Drawing for the job (mm, zero at the part's lowest x, y, z). Give positions to 0.01 mm unless a question says otherwise; leave off trailing zeros. Order: outer loops, then holes, each group sorted by start corner. A loop starts at its lowest first (then second) coordinate and runs counter-clockwise, first axis right, second up. Notation, with made-up numbers: (53, -15.75) - (59, -15.75) arc R7 ccw to (59, -10.75) - close; hole circle Ø5 at (-32.75, -1.75). An arc over 180 degrees is marked (long way). One line per item, written item: value.
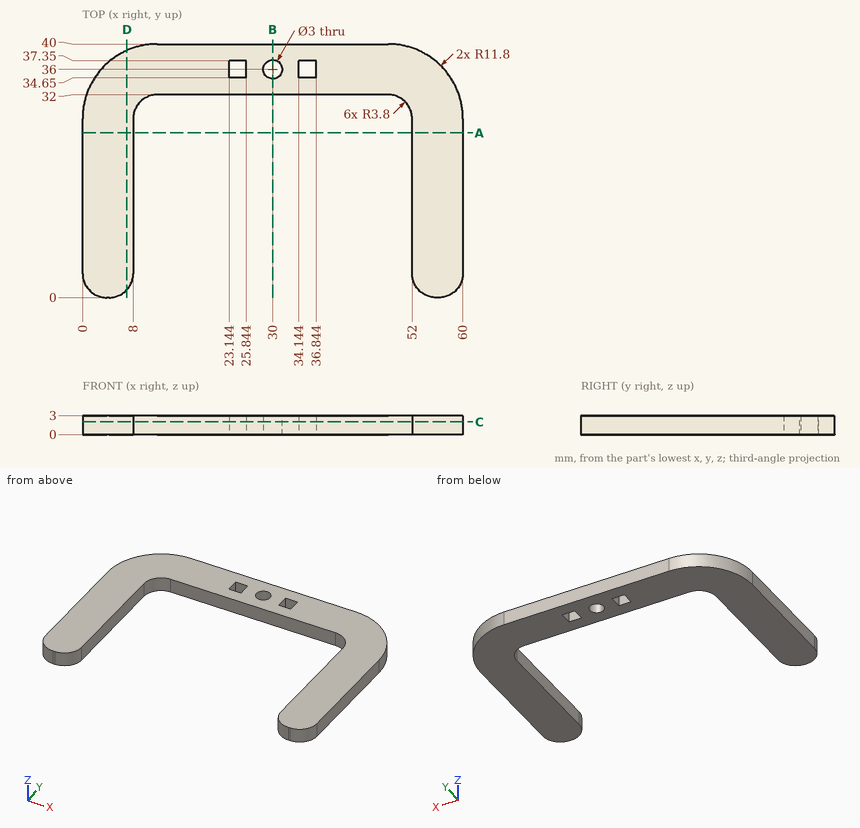
1) Cut at B-B, the plane x = 30. Give the cut face in (y, z).
Outcome:
outline: (32, 0) - (34.5, 0) - (34.5, 3) - (32, 3) - close; (37.5, 0) - (40, 0) - (40, 3) - (37.5, 3) - close
2) Cut at D-D, the plane x = 7. Give the cut face in (y, z).
Outcome:
outline: (1.23, 0) - (38.98, 0) - (38.98, 3) - (1.23, 3) - close
3) Cut at C-C, the plane z = 2. Give the number of separate pieces and of enclosed holes in the cut face.
Outcome:
separate pieces: 1
enclosed holes: 3
4) Drill centre lines: line 1 along Y through (x, z) = (30, 1.6); line 2 along X through (y, z) = (23.5, 1.8); line 3 along X through (y, z) = (36, 2.3) (1 decimal). Where is each one in solid material? Low to high. Write a range as from..to.
Outcome:
line 1: y = 32..34.5, 37.5..40
line 2: x = 0..8, 52..60
line 3: x = 2.9..23.1, 25.8..28.5, 31.5..34.1, 36.8..57.1
5) Cut at A-A, the plane y = 26. Give the cut face in (x, z).
Outcome:
outline: (0, 0) - (8, 0) - (8, 3) - (0, 3) - close; (52, 0) - (60, 0) - (60, 3) - (52, 3) - close
6) Pin check, flat tips, straight feed: pin 1 (0.8 mm diameter, centred on y = 35.5, z = 2, fed in from +X); pin 2 (1.5 mm diameter, centred on x = 23.5, z = 1.5, fed in from -Y); pin 3 (1.4 mm diameter, centred on y = 35.5, z = 1.5, fed in from +X). Stop position of each tip, or through.
Outcome:
pin 1: stops at x = 57.77
pin 2: stops at y = 32
pin 3: stops at x = 57.98
